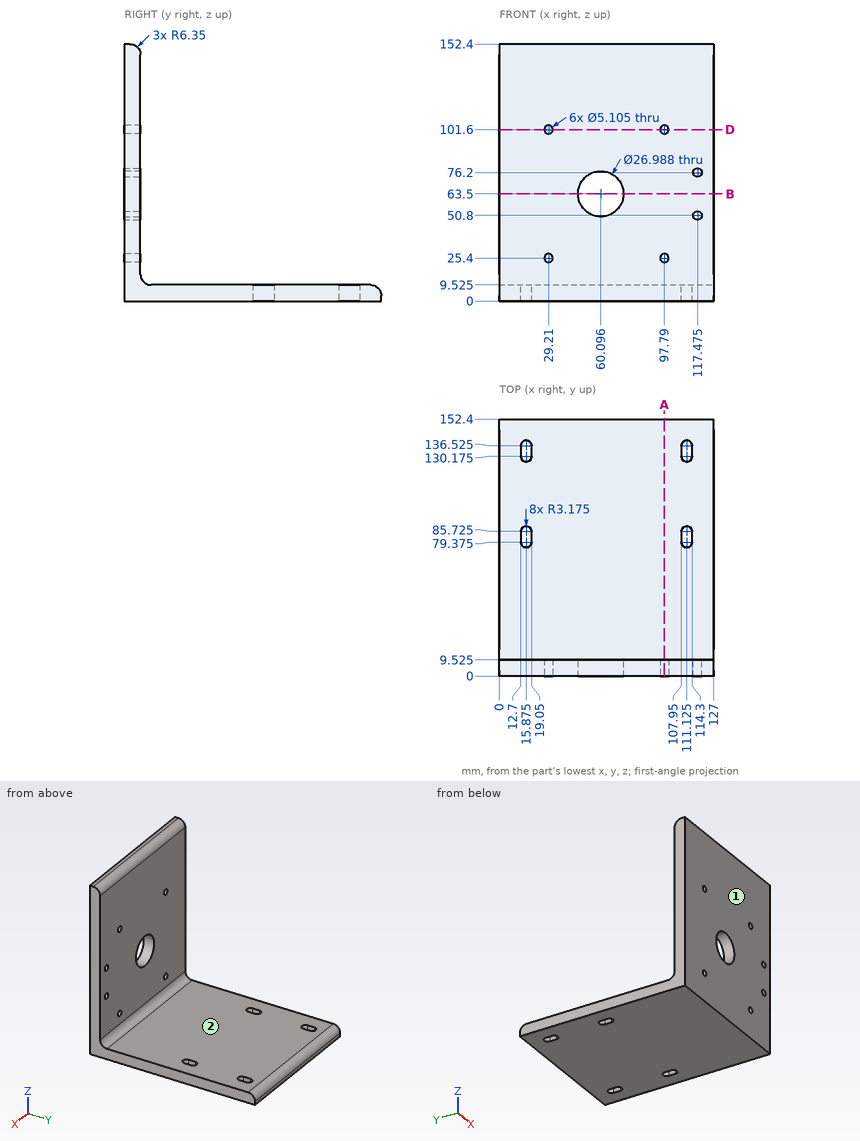
For this review, use the dimensioned drawing (mm, ordinates from the lowest corner) and the shaded views. A direction names the side the tool comes from. Round coordinates to 2 decimals unless told otherwise and drop trailing zeros. Order: outer loops, then holes, each group sorted by start corner. A loop starts at its lowest first (then second) coordinate and runs counter-clockwise, first axis right, second up. Notation, with made-up numbers: M 3,31.25 L 50,31.25 A28 ccw 50,49.25 Z; hole C 86,4 d4. An arc over 180 degrees is marked long. Use a Markdown table: item, result.
1) Wall thickness on line 1 along Z through (x, y) = (29.21, 2.5); line 2 along X through (y, z) = (3, 101.6); line 3 along Z through (x, y) = (28.5, 105) (1 decimal): over which ranges is each line inside the solid? List them lowest first. Write a range as [from, to].
Report:
| item | result |
|---|---|
| line 1 | [0, 22.85], [27.95, 99.05], [104.15, 152.4] |
| line 2 | [0, 26.66], [31.76, 95.24], [100.34, 127] |
| line 3 | [0, 9.5] |
2) Consider section D-D (z = 101.6). Write out the cut boundary in (x, y) (1 decimal), then the cut area to 3 significant figures.
Report:
| item | result |
|---|---|
| outline | M 0,0 L 26.7,0 L 26.7,9.5 L 0,9.5 Z; M 31.8,0 L 95.2,0 L 95.2,9.5 L 31.8,9.5 Z; M 100.3,0 L 127,0 L 127,9.5 L 100.3,9.5 Z |
| area | 1,110 mm^2 |
3) Insertion check: pin 1 (8 mm diameter, centred on x = 112, z = 71, fed in from +Y) (1 decimal); pin 2 (10 mm diameter, centred on x = 94.5, y = 15.5, fed in from +Z) (1 decimal); pin 3 (4.5 mm diameter, centred on x = 117.475, z = 50.8, fed in from -Y); pin 4 (5 mm diameter, centred on x = 20, y = 118.5, fed in from +Z) (1 decimal). Each pin has a flat end and moves straight along its axis. Give the tip position at first contact, or say it passes through.
Report:
| item | result |
|---|---|
| pin 1 | y = 9.5 |
| pin 2 | z = 12.5 |
| pin 3 | through |
| pin 4 | z = 9.5 |
4) Consider section A-A (x = 97.79). Give the number of separate pieces and of enclosed holes in the cut face, then the cut area to 3 significant figures.
Report:
| item | result |
|---|---|
| separate pieces | 3 |
| enclosed holes | 0 |
| area | 2,710 mm^2 |
5) Tool access review of the marked faces 1 and 2: name each direction out of +Z, -Z, +X, -X, +Y, -Y from which nothing blocks a thin tool from reaching the whole face with its end or side.
Report:
| item | result |
|---|---|
| face 1 | +Z, -Z, +X, -X, -Y |
| face 2 | +Z, +X, -X, +Y |
6) Consider section B-B (z = 63.5). Write out the cut boundary in (x, y) (1 decimal).
Report:
| item | result |
|---|---|
| outline | M 0,0 L 46.6,0 L 46.6,9.5 L 0,9.5 Z; M 73.6,0 L 127,0 L 127,9.5 L 73.6,9.5 Z |
